```python
from build123d import *

# Parameters (mm, degrees)
SKETCH1_R               = 35
SKETCH1_R_2             = 12.5
BOSS_EXTRUDE2_DEPTH     = 3
FILLET1_R               = 2
CUT_EXTRUDE1_DEPTH      = 50.859803449
CUT_EXTRUDE1_DEPTH_BACK = 50.859803449
CIRPATTERN4_COUNT       = 10


with BuildPart() as part:
    # Sketch1 → Boss-Extrude2 (new, symmetric)
    with BuildSketch(Plane.XY):
        Circle(SKETCH1_R)
        with BuildLine():
            ThreePointArc((-8.256095748, 9.385461256), (-6.25, 10.825317547), (-4, 11.842719282))
            Line((-4, 11.842719282), (-6, 21.685248442))
            ThreePointArc((-6, 21.685248442), (0, 22.5), (6, 21.685248442))
            Line((6, 21.685248442), (4, 11.842719282))
            ThreePointArc((4, 11.842719282), (6.25, 10.825317547), (8.256095748, 9.385461256))
            Line((8.256095748, 9.385461256), (15.779976038, 16.038776644))
            ThreePointArc((15.779976038, 16.038776644), (19.485571585, 11.25), (21.779976038, 5.646471798))
            Line((21.779976038, 5.646471798), (12.256095748, 2.457258026))
            ThreePointArc((12.256095748, 2.457258026), (12.438874484, 1.234666584), (12.5, 0))
            ThreePointArc((12.5, 0), (12.438874484, -1.234666584), (12.256095748, -2.457258026))
            Line((12.256095748, -2.457258026), (21.779976038, -5.646471798))
            ThreePointArc((21.779976038, -5.646471798), (19.485571585, -11.25), (15.779976038, -16.038776644))
            Line((15.779976038, -16.038776644), (8.256095748, -9.385461256))
            ThreePointArc((8.256095748, -9.385461256), (6.25, -10.825317547), (4, -11.842719282))
            Line((4, -11.842719282), (6, -21.685248442))
            ThreePointArc((6, -21.685248442), (0, -22.5), (-6, -21.685248442))
            Line((-6, -21.685248442), (-4, -11.842719282))
            ThreePointArc((-4, -11.842719282), (-6.25, -10.825317547), (-8.256095748, -9.385461256))
            Line((-8.256095748, -9.385461256), (-15.779976038, -16.038776644))
            ThreePointArc((-15.779976038, -16.038776644), (-19.485571585, -11.25), (-21.779976038, -5.646471798))
            Line((-21.779976038, -5.646471798), (-12.256095748, -2.457258026))
            ThreePointArc((-12.256095748, -2.457258026), (-12.5, 0), (-12.256095748, 2.457258026))
            Line((-12.256095748, 2.457258026), (-21.779976038, 5.646471798))
            ThreePointArc((-21.779976038, 5.646471798), (-19.485571585, 11.25), (-15.779976038, 16.038776644))
            Line((-15.779976038, 16.038776644), (-8.256095748, 9.385461256))
        make_face(mode=Mode.SUBTRACT)
        Circle(SKETCH1_R_2)
    extrude(amount=BOSS_EXTRUDE2_DEPTH, both=True)

    # Fillet1
    fillet1_edges = [part.edges().sort_by_distance(p)[0] for p in [
        (8.256095748, -9.385461256, 0),
        (15.779976038, -16.038776644, 0),
        (21.779976038, -5.646471798, 0),
        (12.256095748, -2.457258026, 0),
        (-6, -21.685248442, 0),
        (6, -21.685248442, 0),
        (4, -11.842719282, 0),
        (-4, -11.842719282, 0),
        (-21.779976038, -5.646471798, 0),
        (-15.779976038, -16.038776644, 0),
        (-8.256095748, -9.385461256, 0),
        (-12.256095748, -2.457258026, 0),
        (-15.779976038, 16.038776644, 0),
        (-21.779976038, 5.646471798, 0),
        (-12.256095748, 2.457258026, 0),
        (-8.256095748, 9.385461256, 0),
        (6, 21.685248442, 0),
        (-6, 21.685248442, 0),
        (-4, 11.842719282, 0),
        (4, 11.842719282, 0),
        (21.779976038, 5.646471798, 0),
        (15.779976038, 16.038776644, 0),
        (8.256095748, 9.385461256, 0),
        (12.256095748, 2.457258026, 0),
    ]]
    fillet(fillet1_edges, radius=FILLET1_R)

    # Sketch4 → Cut-Extrude1 (cut, two sides)
    with BuildSketch(Plane(origin=(0, 0, -3), x_dir=(-1, 0, 0), z_dir=(0, 0, -1))) as cut_extrude1_sk:
        with BuildLine():
            Line((-1.1, 1.161895004), (-1.1, -1.161895004))
            ThreePointArc((-1.1, -1.161895004), (1.6, 0), (-1.1, 1.161895004))
        make_face()
    extrude(amount=CUT_EXTRUDE1_DEPTH, mode=Mode.SUBTRACT)
    extrude(cut_extrude1_sk.sketch, amount=-CUT_EXTRUDE1_DEPTH_BACK, mode=Mode.SUBTRACT)

    # Sketch6 → Ø5.0mm Dowel Hole1 (revolve, cut)
    with BuildSketch(Plane(origin=(0, 30, 3), x_dir=(0, -1, 0), z_dir=(1, 0, 0))):
        Polygon((0, 0), (0, 21.351936393), (2.25, 20), (2.25, 0.275), (2.525, 0), align=None)
    f_5_0mm_dowel_hole1 = revolve(axis=Axis((0, 30, 9.35), (0, 0, -1)), mode=Mode.SUBTRACT)

    # CirPattern4: Ø5.0mm Dowel Hole1 ×10 about axis
    cirpattern4_axis = Axis((0, 0, 0), (0, 0, 1))
    for i in range(1, CIRPATTERN4_COUNT):
        add(f_5_0mm_dowel_hole1.rotate(cirpattern4_axis, i * 360 / CIRPATTERN4_COUNT), mode=Mode.SUBTRACT)


solid = part.part
```
Geometry: final body of the model. Coordinates: model frame, mm. A direction names the side the tool comes from. Round coordinates to 2 decimals unless told otherwise and drop trailing zeros. Order: outer loops, then holes, each group sorted by start corner. A loop starts at its lowest first (then second) coordinate and runs counter-clockwise, first axis right, second up. Notation, with made-up numbers: (2.25, -33) -> (50.25, -33) arc R33 cw to (50.25, 3) -> close; hole circle Ø5 at (46.25, -22). An arc over 180 degrees is marked (long way). Use one line per item in the form item = value. Start each with the question number.
1. Cut plane D-D (z = -0.05). Count the separate pieces of the cut face and the enclosed holes in it, then the cut area to 3 significant figures.
2. Cut plane B-B (y = 0). Return the cut outline in (x, z), then the cut area to 3 significant figures.
3. Draft query along Y for faces 3 (the face through (7, 0, -3)), 4 (the face through (-5.02, -16.87, 0.04)), 5 (the face through (-17.04, 4.06, 0.04)). Return one class per face: pulls with the +Y half, pulls with the -Y half, needs draft (parallel to the pull), parting line crosses it, or undercut.
4. Cut plane A-A (x = 0). Return the cut outline in (y, z) (3 decimals).
5. Reachability of faces 1 (the face through (7, 0, 3)), 2 (the face through (-9.155, -9.447, 0.042)) from +Z, -Z, +X, -X, +Y, -Y: full face, straight path, thin tool, end or side. Return the list, or none.
6. Cut plane C-C (y = -30). Return the cut outline in (x, z) (3 decimals).
7. Pin query (flat end, axial travel): pin 1 Ø5 at (x, y) = (0, -30) entering from +Z (3 decimals); pin 2 Ø3 at (y, z) = (-5.5, -1) entering from -X; pin 3 Ø1.5 at (x, z) = (-25, -1.5) entering from -Y. Return the tip coordinate at first contact, or that it passes through.
8. Line query: probe 1 along Y at (x, z) = (0, 0); probe 2 along X at (y, z) = (6, 2.8); probe 3 along Y at (x, z) = (13, 1.1). Output: solid intervals per line, ascending.
Solution:
q1.separate_pieces = 1
q1.enclosed_holes = 17
q1.area = 3,090 mm^2
q2.outline = (-35, -3) -> (-1.6, -3) -> (-1.6, 3) -> (-35, 3) -> close; (1.1, -3) -> (35, -3) -> (35, 3) -> (1.1, 3) -> close
q2.area = 404 mm^2
q3.face_3 = needs draft
q3.face_4 = undercut
q3.face_5 = undercut
q4.outline = (-35, -3) -> (-32.25, -3) -> (-32.25, 2.725) -> (-32.525, 3) -> (-35, 3) -> close; (-27.75, -3) -> (-22.5, -3) -> (-22.5, 3) -> (-27.475, 3) -> (-27.75, 2.725) -> close; (-12.5, -3) -> (-1.6, -3) -> (-1.6, 3) -> (-12.5, 3) -> close; (1.6, -3) -> (12.5, -3) -> (12.5, 3) -> (1.6, 3) -> close; (22.5, -3) -> (27.75, -3) -> (27.75, 2.725) -> (27.475, 3) -> (22.5, 3) -> close; (32.25, -3) -> (35, -3) -> (35, 3) -> (32.525, 3) -> (32.25, 2.725) -> close
q5.face_1 = +Z, +X, -X, +Y, -Y
q5.face_2 = +Z, -Z
q6.outline = (-18.028, -3) -> (-2.25, -3) -> (-2.25, 2.725) -> (-2.525, 3) -> (-18.028, 3) -> close; (2.25, -3) -> (18.028, -3) -> (18.028, 3) -> (2.525, 3) -> (2.25, 2.725) -> close
q7.pin_1 = 2.975
q7.pin_2 = -34.77
q7.pin_3 = -25.24
q8.probe_1 = -35 to -32.25, -27.75 to -22.5, -12.5 to -1.6, 1.6 to 12.5, 22.5 to 27.75, 32.25 to 35
q8.probe_2 = -34.48 to -21.07, -10.97 to 10.97, 21.07 to 34.48
q8.probe_3 = -32.5 to -13.58, -3.11 to 3.11, 13.58 to 32.5
